```python
from build123d import *

# Parameters (mm, degrees)
BOSS_EXTRUDE1_DEPTH                                 = 20.32
CBORE_FOR_0_BINDING_HEAD_MACHINE_SCREW1_D           = 6.35
CBORE_FOR_0_BINDING_HEAD_MACHINE_SCREW1_CBORE_D     = 8.89
CBORE_FOR_0_BINDING_HEAD_MACHINE_SCREW1_CBORE_DEPTH = 16.51
CUT_EXTRUDE1_DEPTH                                  = 42.890753156
CUT_EXTRUDE1_DEPTH_BACK                             = 42.890753156
SKETCH5_R                                           = 1.905
SKETCH6_R                                           = 2.54
CUT_EXTRUDE2_DEPTH                                  = 7.62
CUT_EXTRUDE3_DEPTH                                  = 7.62


with BuildPart() as part:
    # Sketch1 → Boss-Extrude1 (new body)
    with BuildSketch(Plane.XY):
        Polygon((0, 0), (0, 12.7), (2.54, 12.7), (2.54, 20.32), (27.94, 20.32), (27.94, 12.7), (30.48, 12.7), (30.48, 0), align=None)
    extrude(amount=-BOSS_EXTRUDE1_DEPTH)

    # CBORE for #0 Binding Head Machine Screw1 (through all)
    with Locations(Plane(origin=(0, 0, -20.32), x_dir=(-1, 0, 0), z_dir=(0, 0, -1))):
        with Locations((-15.24, 7.62)):
            CounterBoreHole(CBORE_FOR_0_BINDING_HEAD_MACHINE_SCREW1_D / 2, CBORE_FOR_0_BINDING_HEAD_MACHINE_SCREW1_CBORE_D / 2, CBORE_FOR_0_BINDING_HEAD_MACHINE_SCREW1_CBORE_DEPTH)

    # Sketch5 → Cut-Extrude1 (cut, two sides: drawn at the far end of the back side and taken through both)
    with BuildSketch(Plane(origin=(0, 20.32, 0), x_dir=(1, 0, 0), z_dir=(0, 1, 0)).offset(-CUT_EXTRUDE1_DEPTH_BACK)):
        with Locations(Location((6.35, 6.35, 0), (0, 0, 270))):
            Circle(SKETCH5_R)
        with Locations(Location((24.13, 6.35, 0), (0, 0, 270))):
            Circle(SKETCH5_R)
    extrude(amount=CUT_EXTRUDE1_DEPTH + CUT_EXTRUDE1_DEPTH_BACK, mode=Mode.SUBTRACT)

    # Sketch6 → Cut-Extrude2 (cut)
    with BuildSketch(Plane(origin=(0, 20.32, 0), x_dir=(1, 0, 0), z_dir=(0, 1, 0))):
        with Locations(Location((15.24, 6.35, 0), (0, 0, 270))):
            Circle(SKETCH6_R)
    extrude(amount=-CUT_EXTRUDE2_DEPTH, mode=Mode.SUBTRACT)

    # Sketch7 → Cut-Extrude3 (cut)
    with BuildSketch(Plane.XZ):
        Polygon((1.950590949, -6.35), (4.150295474, -10.16), (8.549704526, -10.16), (10.749409051, -6.35), (8.549704526, -2.54), (4.150295474, -2.54), align=None)
        Polygon((19.730590949, -6.35), (21.930295474, -10.16), (26.329704526, -10.16), (28.529409051, -6.35), (26.329704526, -2.54), (21.930295474, -2.54), align=None)
    extrude(amount=-CUT_EXTRUDE3_DEPTH, mode=Mode.SUBTRACT)


solid = part.part
```
Source: CAD feature listing. Evaluate the final solid. Frame: model axes, mm. A direction names the side the tool comes from. Give positions to 0.01 mm unless a question says otherwise; leave off trailing zeros. Loops run counter-clockwise (first coordinate to the right, second up) from the corner with the lowest first, then second, coordinate; pieces in that order, holes last. Notation, with made-up numbers: (22.5, -1.75) - (36.5, -1.75) arc R8 cw to (36.5, 7.25) - close; hole circle Ø2 at (52.25, 29). An arc over 180 degrees is marked (long way). Use CSV: the item, a comma, the result in double quotes. Start each with the question number.
1. Pin query (flat end, axial travel): pin 1 (1.3 mm diameter, centred on x = 6.5, y = 2, fed in from +Z); pin 2 (2.5 mm diameter, centred on y = 17.5, z = -6, fed in from +X); pin 3 (3 mm diameter, centred on x = 15.24, z = -6.35, fed in from +Y); pin 4 (4 mm diameter, centred on y = 17, z = -12.5, fed in from -X). Return the tip coordinate at first contact, or that it passes through.
2. Ray query, L1, parallel to X at y = 17.75, z = -6.35 (3 decimals); L2, parallel to Z at x = 6.35, y = 16.75 (3 decimals); L3, parallel to X at y = 11, z = -6.35 (3 decimals). Return the intervals inside material, ascending.
3. Section C-C (z = -12.25). Output: boundary loops of the cut face in (x, y) (3 decimals), then the cut area to 3 significant figures.
4. Section B-B (y = 16). Output: boundary loops of the cut face in (x, z) (3 decimals), then the cut area to 3 significant figures.
5. Section A-A (x = 6.35). Output: boundary loops of the cut face in (y, z) (3 decimals), then the cut area to 3 significant figures.
6. Reachability of faces 4 (the flat face through (29, 12.7, -10)), 5 (the flat face through (15, 12.7, -6)), 6 (the flat face through (0, 6, -10)), 7 (the flat face through (27.414, 3.757, -8.282)), 8 (the flat face through (2.54, 16, -10)) from +Z, -Z, +X, -X, +Y, -Y: full face, straight path, thin tool, end or side. Return the list, or none.
7. Section D-D (x = 15.24). Output: boundary loops of the cut face in (y, z) (3 decimals).
8. Draft query along Z for faces 1 (the flat face through (26, 7.62, -5)), 2 (the flat face through (15, 13, -20.32)), 3 (the flat face through (15, 0, -10)). Return one class per face: +Z half, -Z half, draft (parallel to the pull), parting line (faces both ways), or undercut.
Response:
1,pin 1,"z = 0"
1,pin 2,"x = 27.94"
1,pin 3,"y = 12.7"
1,pin 4,"x = 2.54"
2,L1,"2.54 to 4.445, 8.255 to 12.7, 17.78 to 22.225, 26.035 to 27.94"
2,L2,"-20.32 to -8.255, -4.445 to 0"
2,L3,"0 to 4.445, 8.255 to 12.353, 18.127 to 22.225, 26.035 to 30.48"
3,outline,"(0, 0) - (30.48, 0) - (30.48, 12.7) - (27.94, 12.7) - (27.94, 20.32) - (2.54, 20.32) - (2.54, 12.7) - (0, 12.7) - close; hole circle Ø8.89 at (15.24, 7.62)"
3,area,"519 mm²"
4,outline,"(2.54, -20.32) - (27.94, -20.32) - (27.94, 0) - (2.54, 0) - close; hole circle Ø3.81 at (6.35, -6.35); hole circle Ø5.08 at (15.24, -6.35); hole circle Ø3.81 at (24.13, -6.35)"
4,area,"473 mm²"
5,outline,"(0, -20.32) - (20.32, -20.32) - (20.32, -8.255) - (7.62, -8.255) - (7.62, -10.16) - (0, -10.16) - close; (0, -2.54) - (7.62, -2.54) - (7.62, -4.445) - (20.32, -4.445) - (20.32, 0) - (0, 0) - close"
5,area,"306 mm²"
6,face 4,"+Z, -Z, +X, +Y"
6,face 5,"+Y"
6,face 6,"+Z, -Z, -X, +Y, -Y"
6,face 7,"-Y"
6,face 8,"+Z, -Z, -X, +Y"
7,outline,"(0, -20.32) - (3.175, -20.32) - (3.175, -3.81) - (4.445, -3.81) - (4.445, 0) - (0, 0) - close; (10.795, -3.81) - (12.065, -3.81) - (12.065, -20.32) - (20.32, -20.32) - (20.32, -8.89) - (12.7, -8.89) - (12.7, -3.81) - (20.32, -3.81) - (20.32, 0) - (10.795, 0) - close"
8,face 1,"undercut"
8,face 2,"-Z half"
8,face 3,"draft"
